The figure shows three views and two pictorial views of one solid part (mm, origin at its lowest corner). Answer the questions. Coordinates: 2 decimals unless noted, no trailing zeros. Write each loop counter-clockwise with the first axis right and the second up, starting at its lowest first coordinate (ties: lowest second). Pieces come first, ordered by that corner, then holes.
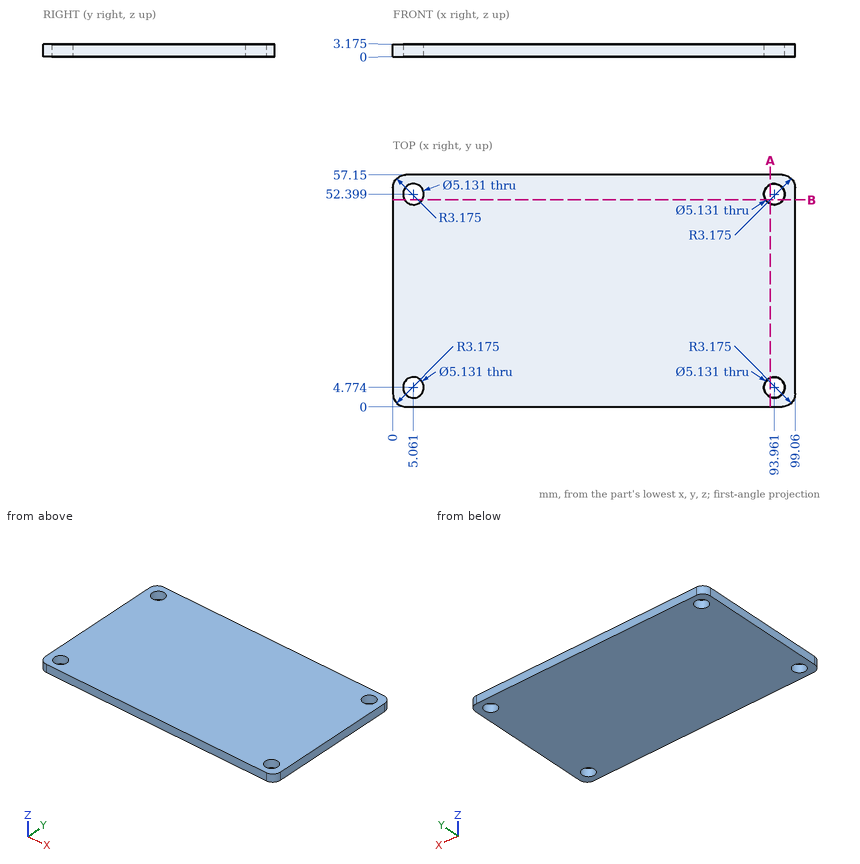
1. Find the intervals of material crossed by L1, parallel to X at y = 7, z = 2 (1 decimal); L2, parallel to X at y = 3, z = 0.9 (1 decimal), in increasing order.
Results found:
L1: x = 0 to 3.8, 6.3 to 92.7, 95.2 to 99.1
L2: x = 0 to 3.2, 6.9 to 92.1, 95.8 to 99.1
2. Section B-B on y = 51 is taken. Give the vertices of the cut face in (x, z) (1 decimal).
Results found:
outline: (0, 0) - (2.9, 0) - (2.9, 3.2) - (0, 3.2) - close; (7.2, 0) - (91.8, 0) - (91.8, 3.2) - (7.2, 3.2) - close; (96.1, 0) - (99.1, 0) - (99.1, 3.2) - (96.1, 3.2) - close
3. Section A-A on x = 93 is taken. State how many separate pieces and enclosed holes the cut face has, then the cut area to 3 significant figures.
Results found:
separate pieces: 3
enclosed holes: 0
area: 151 mm2
